from build123d import *

# Parameters (mm, degrees)
SKETCH1_W           = 12.538434267
SKETCH1_H           = 35
BOSS_EXTRUDE1_DEPTH = 4
SKETCH2_W           = 2.538434267
SKETCH2_H           = 21
CUT_EXTRUDE1_DEPTH  = 37.619666847
SKETCH3_W           = 2.5
SKETCH3_H           = 21
CUT_EXTRUDE2_DEPTH  = 37.619666847
CUT_EXTRUDE3_DEPTH  = 37.619666847
SKETCH5_W           = 7.5
SKETCH5_H           = 1.65
SKETCH6_W           = 7.5
SKETCH6_H           = 1.65
HOLE1_D             = 2.013
FILLET1_R           = 1.25


with BuildPart() as part:
    # Sketch1 → Boss-Extrude1 (new body)
    with BuildSketch(Plane(origin=(0, 0, 0), x_dir=(-1, 0, 0), z_dir=(0, 0, -1))):
        with Locations((3.730782867, 17.5)):
            Rectangle(SKETCH1_W, SKETCH1_H)
    extrude(amount=-BOSS_EXTRUDE1_DEPTH)

    # Sketch2 → Cut-Extrude1 (cut, through all)
    with BuildSketch(Plane.XY.offset(4)):
        with Locations((1.269217133, 17.5)):
            Rectangle(SKETCH2_W, SKETCH2_H)
    extrude(amount=-CUT_EXTRUDE1_DEPTH, mode=Mode.SUBTRACT)

    # Sketch3 → Cut-Extrude2 (cut, through all)
    with BuildSketch(Plane.XY.offset(4)):
        with Locations((-8.75, 17.5)):
            Rectangle(SKETCH3_W, SKETCH3_H)
    extrude(amount=-CUT_EXTRUDE2_DEPTH, mode=Mode.SUBTRACT)

    # Sketch4 → Cut-Extrude3 (cut, through all)
    with BuildSketch(Plane(origin=(0, 0, 0), x_dir=(0, 0, -1), z_dir=(1, 0, 0))):
        with BuildLine():
            Line((-2.855933763, 23.21436986), (-2.855933763, 11.78563014))
            ThreePointArc((-2.855933763, 11.78563014), (-1.992824856, 12.024984399), (-1.13183027, 11.778132681))
            Line((-1.13183027, 11.778132681), (-1.13183027, 23.221867319))
            ThreePointArc((-1.13183027, 23.221867319), (-1.992824856, 22.975015601), (-2.855933763, 23.21436986))
        make_face()
    extrude(amount=-CUT_EXTRUDE3_DEPTH, mode=Mode.SUBTRACT)

    # Sketch5 → Cut-Revolve1 (revolve, cut)
    with BuildSketch(Plane.XY.offset(2)):
        with Locations((-3.75, 11.2)):
            Rectangle(SKETCH5_W, SKETCH5_H)
    revolve(axis=Axis((-7.5, 10.375, 2), (1, 0, 0)), mode=Mode.SUBTRACT)

    # Sketch6 → Cut-Revolve2 (revolve, cut)
    with BuildSketch(Plane.XY.offset(2)):
        with Locations((-3.75, 25.45)):
            Rectangle(SKETCH6_W, SKETCH6_H)
    revolve(axis=Axis((-7.5, 24.625, 2), (1, 0, 0)), mode=Mode.SUBTRACT)

    # Hole1 (through all)
    with Locations(Plane(origin=(0, 0, 0), x_dir=(-1, 0, 0), z_dir=(0, 0, -1))):
        with Locations((0.730782866, 3.5), (6.730782866, 3.5), (0.730782866, 31.5), (6.730782866, 31.5)):
            Hole(HOLE1_D / 2)

    # Fillet1
    fillet1_edges = [part.edges().sort_by_distance(p)[0] for p in [
        (0, 7, 2),
        (0, 28, 2),
        (-7.5, 28, 2),
        (-7.5, 7, 2),
    ]]
    fillet(fillet1_edges, radius=FILLET1_R)


solid = part.part
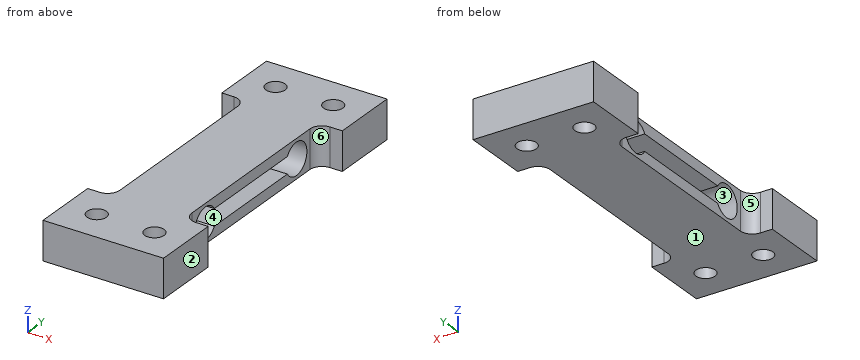
Input: part model. Units: mm. Frame: model coordinates. Face numbers are marked on the shaded views. A direction names the side the tool comes from. Give positions to 0.01 mm unless a question says otherwise; leave off trailing zeros. Write each loop counter-clockwise with the first axis right and the second up, starting at its lowest first coordinate (ties: lowest second). Pieces come first, ordered by that corner, then holes. Notation, with made-up numbers: M -11,-22 L 5,-22 A18 cw 5,-1 Z; hole C 17.5,69 d7. An arc over 180 degrees is marked long. Use one line per item in the form item = value.
1. Cut plane C-C on x = -3.25. Return loops of the section in (y, z) (3 decimals).
Outcome:
outline = M 0,0 L 35,0 L 35,4 L 0,4 Z; hole M 11.778,1.132 L 23.222,1.132 A1.65 ccw long 23.214,2.856 L 11.786,2.856 A1.65 ccw long Z
2. Mould query, pull axis Z, two halves, no side actions, for the marked faces 1, 2 and 3. Classes: released by +Z, released by -Z, zero draft, split by the parting line, or undercut.
Outcome:
face_1 = released by -Z
face_2 = zero draft
face_3 = undercut
3. Reachability of the marked faces 4, 5 and 6 from +Z, -Z, +X, -X, +Y, -Y: full face, straight path, thin tool, end or side. Return the list, or none.
Outcome:
face_4 = +X, -X
face_5 = +Z, -Z, -X
face_6 = +Z, -Z, +X
4. Cut plane D-D on x = -1.25. Return loops of the section in (y, z) (3 decimals), and give its area (3 significant figures).
Outcome:
outline = M 0,0 L 2.638,0 L 2.638,4 L 0,4 Z; M 4.362,0 L 30.638,0 L 30.638,4 L 4.362,4 Z; M 32.362,0 L 35,0 L 35,4 L 32.362,4 Z; hole M 11.778,1.132 L 23.222,1.132 A1.65 ccw long 23.214,2.856 L 11.786,2.856 A1.65 ccw long Z
area = 89.9 mm²
5. Cut plane A-A on z = 2. State how many separate pieces and enclosed holes the cut face has, and give its area (3 significant figures).
Outcome:
separate_pieces = 2
enclosed_holes = 4
area = 190 mm²
6. Ray query, L1, parallel to Y at x = -4, z = 2 (3 decimals); L2, parallel to Z at x = -3.5, y = 23; L3, parallel to Y at x = -2.75, z = 0.7. Return the intervals inside material, ascending.
Outcome:
L1 = 0 to 8.725, 26.275 to 35
L2 = 0 to 1.13, 2.86 to 4
L3 = 0 to 9.36, 11.39 to 23.61, 25.64 to 35
7. First-contact query: P1, Ø1.2, axis at y = 16.5, z = 3, coming from the +X side; P2, Ø1.2, axis at y = 14.5, z = 2.5, coming from the -X side; P3, Ø1, axis at y = 27, z = 1, coming from the -X side. Flat tips, straight axial feed; report the tip coordinate or a pass-through.
Outcome:
P1 = 0
P2 = -7.5
P3 = -7.75
8. Cut plane B-B on y = 21. Return loops of the section in (x, z), and give its area (3 significant figures).
Outcome:
outline = M -7.5,0 L 0,0 L 0,1.13 L -7.5,1.13 Z; M -7.5,2.86 L 0,2.86 L 0,4 L -7.5,4 Z
area = 17.1 mm²
